Model file for the job. Use its own axes, mm. Face numbers are marked on the shaded views. A direction names the side the tool comes from. Round coordinates to 2 decimals unless told otherwise and drop trailing zeros. Write each loop counter-clockwise with the first axis right and the second up, starting at its lowest first coordinate (ties: lowest second). Pieces come first, ordered by that corner, then holes. Notation, with made-up numbers: (37, 88.25) - (56, 88.25) arc R20 ccw to (56, 113.25) - close; hole circle Ø9 at (-25.75, 23.5). An arc over 180 degrees is marked (long way). Answer as a JSON object with one key per item and string values. Group by question number.
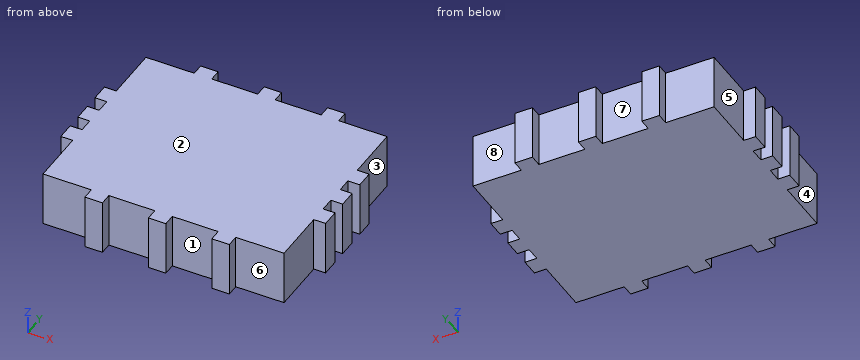
from build123d import *

# Parameters (mm, degrees)
COMPONENT_OUTLINE_DEPTH = 2.2


with BuildPart() as part:
    # 草图1 → Component_Outline (new body)
    with BuildSketch(Plane.XY):
        Polygon((-2.89, -4.3), (-2.89, -3.825), (-4.825, -3.825), (-4.825, -1.62), (-5.3, -1.62), (-5.3, -0.92), (-4.825, -0.92), (-4.825, -0.35), (-5.3, -0.35), (-5.3, 0.35), (-4.825, 0.35), (-4.825, 0.92), (-5.3, 0.92), (-5.3, 1.62), (-4.825, 1.62), (-4.825, 3.825), (-2.89, 3.825), (-2.89, 4.3), (-2.19, 4.3), (-2.19, 3.825), (-0.35, 3.825), (-0.35, 4.3), (0.35, 4.3), (0.35, 3.825), (2.19, 3.825), (2.19, 4.3), (2.89, 4.3), (2.89, 3.825), (4.825, 3.825), (4.825, 1.62), (5.3, 1.62), (5.3, 0.92), (4.825, 0.92), (4.825, 0.35), (5.3, 0.35), (5.3, -0.35), (4.825, -0.35), (4.825, -0.92), (5.3, -0.92), (5.3, -1.62), (4.825, -1.62), (4.825, -3.825), (2.89, -3.825), (2.89, -4.3), (2.19, -4.3), (2.19, -3.825), (0.35, -3.825), (0.35, -4.3), (-0.35, -4.3), (-0.35, -3.825), (-2.19, -3.825), (-2.19, -4.3), align=None)
    extrude(amount=COMPONENT_OUTLINE_DEPTH)


solid = part.part
(1) Slice it at A-A (y = -1.75). Write the cut outline in (x, z) (3 decimals), then the cut area to 3 significant figures.
(2) 3-axis set-ups, long thin cutter, end or side, ignore diameter. For the marked faces 4, 5, 6, 7 and 8: which of +Z, -Z, +X, -X, +Y, -Y reach the whole face in a straight line?
(3) Flat gauge pins, fed straight in: pin 1 (0.5 mm diameter, centred on y = -4, z = 0.5, fed in from +X) (3 decimals); pin 2 (0.5 mm diameter, centred on y = -0.5, z = 1, fed in from -X); pin 3 (0.7 mm diameter, centred on y = 2.5, z = 1, fed in from -X) (3 decimals); pin 4 (0.9 mm diameter, centred on x = 1, z = 0.5, fed in from +Y) (3 decimals). Where does each tip first touch, or does it go through?
(4) Pull direction X, two halves, no side cores. Call the marked faces 1, 2 and 3: pulls with the +X half, pulls with the -X half, needs draft (parallel to the pull), parting line crosses it, or undercut.
(5) Drill centre lines: line 1 (X direction, y = 0.75, z = 0.6) (3 decimals); line 2 (Y direction, x = 3.5, z = 1.7) (3 decimals). Where is each one in solid material? Low to high. Write a range as from..to.
(6) Slice it at B-B (x = -1.75). Write the cut outline in (y, z) (3 decimals), then the cut area to 3 significant figures.
Answer:
{
 "1": {"outline": "(-4.825, 0) - (4.825, 0) - (4.825, 2.2) - (-4.825, 2.2) - close", "area": "21.2 mm²"},
 "2": {"face 4": "+Z, -Z, -X, -Y", "face 5": "+Z, -Z, -X, +Y", "face 6": "+Z, -Z, +X, -Y", "face 7": "+Z, -Z, +Y", "face 8": "+Z, -Z, +X, +Y"},
 "3": {"pin 1": "x = 4.825", "pin 2": "x = -5.3", "pin 3": "x = -4.825", "pin 4": "y = 3.825"},
 "4": {"face 1": "undercut", "face 2": "needs draft", "face 3": "pulls with the +X half"},
 "5": {"line 1": "-4.825..4.825", "line 2": "-3.825..3.825"},
 "6": {"outline": "(-3.825, 0) - (3.825, 0) - (3.825, 2.2) - (-3.825, 2.2) - close", "area": "16.8 mm²"}
}
